Could you check a few things on this model? Use its own coordinates, in mm. Face numbers are marked on the shaded views. Coordinates: 2 decimals unless noted, no trailing zeros. Write each loop counter-clockwise with the first axis right and the second up, starting at its lowest first coordinate (ties: lowest second). Pieces come first, ordered by that corner, then holes.
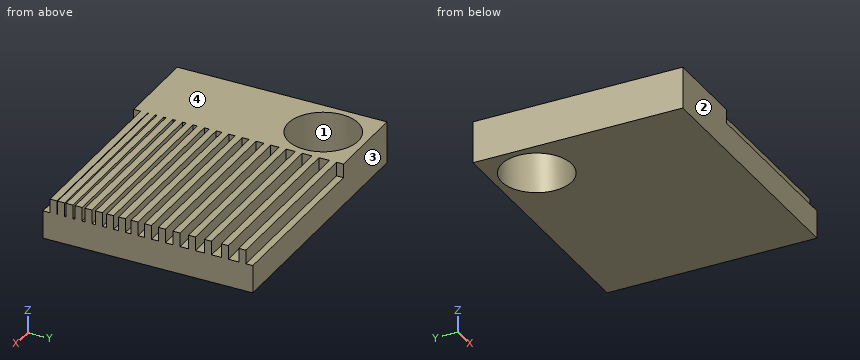
Autodesk Fusion 360 part; units mm, degrees
sketch "Sketch1" plane through (0, 0, 0) normal (0, 0, 1) x (1, 0, 0)
  line L0 (0, 0) -> (37, 0)
  line L1 (37, 0) -> (37, 30)
  line L2 (37, 30) -> (0, 30)
  line L3 (0, 30) -> (0, 0)
  line L4 (12, 30) -> (12, 0) construction
  line L5 (12, 1) -> (37, 1)
  line L6 (12, 2) -> (37, 2)
  line L7 (12, 2.1) -> (37, 2.1)
  line L8 (12, 3.1) -> (37, 3.1)
  line L9 (12, 3.3) -> (37, 3.3)
  line L10 (12, 4.3) -> (37, 4.3)
  line L11 (12, 4.6) -> (37, 4.6)
  line L12 (12, 5.6) -> (37, 5.6)
  line L13 (12, 6) -> (37, 6)
  line L14 (12, 7) -> (37, 7)
  line L15 (12, 7.5) -> (37, 7.5)
  line L16 (12, 8.5) -> (37, 8.5)
  line L17 (12, 9.1) -> (37, 9.1)
  line L18 (12, 10.1) -> (37, 10.1)
  line L19 (12, 10.8) -> (37, 10.8)
  line L20 (37, 11.8) -> (12, 11.8)
  line L21 (12, 12.6) -> (37, 12.6)
  line L22 (37, 13.6) -> (12, 13.6)
  line L23 (12, 14.5) -> (37, 14.5)
  line L24 (37, 15.5) -> (12, 15.5)
  line L25 (12, 16.5) -> (37, 16.5)
  line L26 (37, 17.5) -> (12, 17.5)
  line L27 (12, 18.6) -> (37, 18.6)
  line L28 (37, 19.6) -> (12, 19.6)
  line L29 (12, 23.1) -> (37, 23.1)
  line L30 (12, 20.8) -> (37, 20.8)
  line L31 (12, 21.8) -> (37, 21.8)
  line L32 (12, 24.1) -> (37, 24.1)
  line L33 (37, 25.5) -> (12, 25.5)
  line L34 (12, 26.5) -> (37, 26.5)
  line L35 (37, 28) -> (12, 28)
  line L36 (12, 29) -> (37, 29)
  line L37 (12, 30) -> (12, 0)
  circle A0 centre (6, 24) radius 5
  dimension "d4" = 30
  dimension "d5" = 37
  dimension "d6" = 25
  dimension "d11" = 1
  dimension "d12" = 1
  dimension "d13" = 0.1
  dimension "d14" = 1
  dimension "d15" = 0.2
  dimension "d16" = 1
  dimension "d17" = 0.3
  dimension "d18" = 1
  dimension "d19" = 0.4
  dimension "d20" = 1
  dimension "d21" = 0.5
  dimension "d22" = 1
  dimension "d23" = 0.6
  dimension "d24" = 1
  dimension "d25" = 0.7
  dimension "d26" = 1
  dimension "d27" = 0.8
  dimension "d28" = 1
  dimension "d29" = 0.9
  dimension "d30" = 1
  dimension "d31" = 1
  dimension "d32" = 1
  dimension "d33" = 1.1
  dimension "d34" = 1
  dimension "d35" = 1.2
  dimension "d36" = 1
  dimension "d37" = 1.3
  dimension "d38" = 1
  dimension "d39" = 1.4
  dimension "d40" = 1
  dimension "d41" = 1.5
  dimension "d42" = 1
  dimension "d47" = 10
extrude "Extrude5" add sketch "Sketch1" along normal blind 6 contours L0 L2 L3 L37
extrude "Extrude6" add sketch "Sketch1" along normal blind 6 contours L1 L5 L6 L37 | L1 L35 L36 L37 | L1 L7 L8 L37 | L1 L33 L34 L37 | L1 L9 L10 L37 | L1 L29 L32 L37 | L1 L11 L12 L37 | L1 L30 L31 L37 | L1 L13 L14 L37 | L1 L27 L28 L37 | L1 L15 L16 L37 | L1 L25 L26 L37 | L1 L17 L18 L37 | L1 L23 L24 L37 | L1 L19 L20 L37 | L1 L21 L22 L37
extrude "Extrude7" add sketch "Sketch1" along normal blind 4 contours L0 L1 L5 L37 | L1 L2 L36 L37 | L1 L6 L7 L37 | L1 L34 L35 L37 | L1 L8 L9 L37 | L1 L32 L33 L37 | L1 L10 L11 L37 | L1 L29 L31 L37 | L1 L12 L13 L37 | L1 L28 L30 L37 | L1 L14 L15 L37 | L1 L26 L27 L37 | L1 L16 L17 L37 | L1 L24 L25 L37 | L1 L18 L19 L37 | L1 L22 L23 L37 | L1 L20 L21 L37
sketch "Sketch3" plane through (0, 0, 0) normal (0, -1, 0) x (1, 0, 0)
  line L0 (0, 0) -> (37, 0)
  line L1 (37, 0) -> (37, 4)
  line L2 (37, 4) -> (12, 4)
  line L3 (12, 4) -> (12, 6)
  line L4 (12, 6) -> (0, 6)
  line L5 (0, 6) -> (0, 0)
  line L6 (0, 3) -> (37, 3) construction
  line L7 (6, 0) -> (6, 6) construction
  circle A0 centre (6, 3) radius 1.6
  dimension "d60" = 6
  dimension "d61" = 3.2
extrude "Extrude8" [suppressed]
thread "Thread2" [suppressed]
equation "length = 37 mm"
equation "width = 30 mm"
equation "thickness = 6 mm"
equation "d4 = width"
equation "d5 = length"
equation "d6 = comb_length"
equation "comb_length = 25 mm"
equation "comb_height = 2 mm"
equation "comb_width = 1 mm"
equation "comb_spacing = 0.1 mm"
equation "d12 = comb_width"
equation "d13 = comb_spacing"
equation "d14 = comb_width"
equation "d15 = comb_spacing * 2"
equation "d16 = comb_width"
equation "d17 = comb_spacing * 3"
equation "d18 = comb_width"
equation "d19 = comb_spacing * 4"
equation "d20 = comb_width"
equation "d21 = comb_spacing * 5"
equation "d22 = comb_width"
equation "d23 = comb_spacing * 6"
equation "d24 = comb_width"
equation "d25 = comb_spacing * 7"
equation "d26 = comb_width"
equation "d27 = comb_spacing * 8"
equation "d28 = comb_width"
equation "d29 = comb_spacing * 9"
equation "d30 = comb_width"
equation "d31 = comb_spacing * 10"
equation "d32 = comb_width"
equation "d33 = comb_spacing * 11"
equation "d34 = comb_width"
equation "d35 = comb_spacing * 12"
equation "d36 = comb_width"
equation "d37 = comb_spacing * 13"
equation "d38 = comb_width"
equation "d39 = comb_spacing * 14"
equation "d40 = comb_width"
equation "d41 = comb_spacing * 15"
equation "d42 = comb_width"
equation "d54 = thickness"
equation "d56 = thickness"
equation "d58 = thickness - comb_height"
1. If we mould it in two halves opening along Y, with no side actions, what happens to the marked faces 1, 2, 3 and 4? For each: pulls with the +Y half, pulls with the -Y half, needs draft (parallel to the pull), parting line crosses it, or undercut.
Verdict:
face 1: undercut
face 2: pulls with the -Y half
face 3: pulls with the +Y half
face 4: needs draft
2. I want a section at A-A on x = 6. Please give me the cut outline in (y, z), plus the area to 3 significant figures.
Verdict:
outline: (0, 0) - (19, 0) - (19, 6) - (0, 6) - close; (29, 0) - (30, 0) - (30, 6) - (29, 6) - close
area: 120 mm2
3. I want a section at B-B on z = 1.35. Please give me the cut outline in (x, y), plus the area to 3 significant figures.
Verdict:
outline: (0, 0) - (37, 0) - (37, 30) - (0, 30) - close; hole circle Ø10 at (6, 24)
area: 1,030 mm2
4. Please list where these lines run through material, in increasing order: line 1 along Y through (x, z) = (6, 4); line 2 along Z through (x, y) = (20, 22); line 3 along X through (y, z) = (22, 4.5).
Verdict:
line 1: y = 0 to 19, 29 to 30
line 2: z = 0 to 4
line 3: x = 0 to 1.42, 10.58 to 12
5. For pin 1 (1.6 mm diameter, centred on x = 18.5, z = 5.5, fed in from -Y); pin 2 (1 mm diameter, centred on x = 23, z = 5.5, fed in from +Y); pin 3 (0.8 mm diameter, centred on x = 22, y = 0.5, fed in from +Z), each with a flat end and sliding along its axis, tell me the tip position at first contact or that it passes through.
Verdict:
pin 1: stops at y = 1
pin 2: stops at y = 29
pin 3: stops at z = 4
